from build123d import *

# Parameters (mm, degrees)
BASE_FLANGE2_DEPTH   = 1.5875
M4_CLEARANCE_HOLE1_D = 4.5


# Read off the part's stored shape, not the designer's step: Base-Flange2
with BuildPart() as part:
    # Base-Flange2 outline → Base-Flange2 (new body)
    with BuildSketch(Plane(origin=(0, 0, 0), x_dir=(-1, 0, 0), z_dir=(0, 0, -1))):
        with BuildLine():
            Line((69.65, -9.525), (69.65, 7))
            ThreePointArc((69.65, 7), (62.15, 14.5), (54.65, 7))
            Line((54.65, 7), (54.65, 0))
            Line((54.65, 0), (7.5, 0))
            Line((7.5, 0), (7.5, 7))
            ThreePointArc((7.5, 7), (0, 14.5), (-7.5, 7))
            Line((-7.5, 7), (-7.5, -9.525))
            Line((-7.5, -9.525), (69.65, -9.525))
        make_face()
    extrude(amount=BASE_FLANGE2_DEPTH)

    # M4 Clearance Hole1 (through all)
    with Locations(Plane.XY):
        with Locations((0, 7), (-62.15, 7)):
            Hole(M4_CLEARANCE_HOLE1_D / 2)


solid = part.part
For this review, take the finished solid that the model builds, in its own axes (mm). A direction names the side the tool comes from. Coordinates: 2 decimals unless noted, no trailing zeros. Loops run counter-clockwise (first coordinate to the right, second up) from the corner with the lowest first, then second, coordinate; pieces in that order, holes last. Notation, with made-up numbers: (69, 15) - (107, 15) arc R24 ccw to (107, 36) - close; hole circle Ø1 at (74, -17). An arc over 180 degrees is marked (long way). Use a Markdown table: item, result. Add a question column.
Item 1: Insertion check: pin 1 Ø0.8 at (x, z) = (-27, -1) entering from +Y. The pin has a flat end and moves straight along its axis. Give the tip position at first contact, or say it passes through.
Item 2: Mouldability with a two-part tool opening along Y and no side actions: class faces 1 (the face through (-69.65, -1, -1)), 2 (the face through (-62.3, 14.5, -0.8)), 3 (the face through (-59.902, 7.099, -0.805)), 4 (the face through (-1.21, 8.897, -0.805)) as pulls with the +Y half, pulls with the -Y half, needs draft (parallel to the pull), parting line crosses it, or undercut.
Item 3: For line 1 (X direction, y = 6.5, z = -1.25); line 2 (Y direction, x = 0, z = -0.65) (3 decimals); line 3 (Y direction, x = -53, z = -0.6) (3 decimals), list the stretches that pass through material, from the lowest coordinate up.
Item 4: We need section B-B (z = -0.9). Give the boundary of the cut face in (x, y) (3 decimals), and give its area (3 significant figures).
Item 5: Tool access review of faces 5 (the face through (-31, -3, 0)), 6 (the face through (-54.65, 4, -1)): name each direction out of +Z, -Z, +X, -X, +Y, -Y from which nothing blocks a thin tool from reaching the whole face with its end or side.
Item 6: We need section C-C (y = 12). Give the boundary of the cut face in (x, z).
Item 7: We need section D-D (x = -42.5). Give the boundary of the cut face in (y, z) (1 decimal), and give its area (3 significant figures).
Results list:
| question | item | result |
|---|---|---|
| 1 | pin 1 | stops at y = 0 |
| 2 | face 1 | needs draft |
| 2 | face 2 | pulls with the +Y half |
| 2 | face 3 | undercut |
| 2 | face 4 | undercut |
| 3 | line 1 | x = -69.65 to -64.34, -59.96 to -54.65, -7.5 to -2.19, 2.19 to 7.5 |
| 3 | line 2 | y = -9.525 to 4.75, 9.25 to 14.5 |
| 3 | line 3 | y = -9.525 to 0 |
| 4 | outline | (-69.65, -9.525) - (7.5, -9.525) - (7.5, 7) arc R7.5 ccw to (-7.5, 7) - (-7.5, 0) - (-54.65, 0) - (-54.65, 7) arc R7.5 ccw to (-69.65, 7) - close; hole circle Ø4.5 at (-62.15, 7); hole circle Ø4.5 at (0, 7) |
| 4 | area | 1,090 mm^2 |
| 5 | face 5 | +Z, +X, -X, +Y, -Y |
| 5 | face 6 | +Z, -Z, +Y |
| 6 | outline | (-67.74, -1.59) - (-56.56, -1.59) - (-56.56, 0) - (-67.74, 0) - close; (-5.59, -1.59) - (5.59, -1.59) - (5.59, 0) - (-5.59, 0) - close |
| 7 | outline | (-9.5, -1.6) - (0, -1.6) - (0, 0) - (-9.5, 0) - close |
| 7 | area | 15.1 mm^2 |
